Design review of the part built by this model. Coordinates are the model's own, in mm. Face numbers are marked on the shaded views. A direction names the side the tool comes from. Coordinates: 2 decimals unless noted, no trailing zeros. Loops run counter-clockwise (first coordinate to the right, second up) from the corner with the lowest first, then second, coordinate; pieces in that order, holes last. Notation, with made-up numbers: (84, 47) - (112, 47) arc R27 cw to (112, 64) - close; hole circle Ø2 at (37, 54). An arc over 180 degrees is marked (long way). Answer in a Markdown table with one row per item. Add a question column.
(1) The part is to be moulded in two halves that separate along X. For the marked faces 3, 4 and 5, say which applies: released by +X, released by -X, zero draft, split by the parting line, or undercut.
(2) We need section D-D, the plane x = 1. Write out the cut boundary in (y, z).
(3) We need section A-A, the plane x = 0. Write out the cut boundary in (y, z).
(4) For the marked faces 1 and 2, list the 3-axis set-ups (+Z, -Z, +X, -X, +Y, -Y) from which the entire face can be reached by the end or side of a thin tool; tool diameter is ignored.
(5) Clearance check with flat-ended pins moving along their axes: pin 1 (2.5 mm diameter, centred on x = 1, y = -0.5, fed in from -Z); pin 2 (2 mm diameter, centred on x = 3.5, z = 3, fed in from +Y); pin 3 (1 mm diameter, centred on x = 2.5, z = 1, fed in from +Y). State where each tip first meets the part, or that it passes through.
(6) We need section B-B, the plane y = 0. Write out the cut boundary in (x, z).
(7) To check wall thickness, follow L1, parallel to Y at x = 0, z = 2.2; L2, parallel to Y at x = 0, z = 3.85; L3, parallel to X at y = 0, z = 1.4. State the ranges of each line that lie inside material, in increasing order. Write a range as [from, to].
(8) We need section C-C, the plane z = 3.75. Write out the cut boundary in (x, y).
from build123d import *

# Parameters (mm, degrees)
F0_R     = 4.75
F1_DEPTH = 4
F2_R     = 2
F3_DEPTH = 4
F5_START = -0.75
F4_R     = 2.5
F5_DEPTH = 3.25
F6_W     = 3.7872615503
F6_H     = 0.8450912428
F7_DEPTH = 4


with BuildPart() as f1:
    # F0 (on Top) → F1 (new body)
    with BuildSketch(Plane.XY):
        Circle(F0_R)
    extrude(amount=F1_DEPTH)

    # F2 (on face) → F3 (cut)
    with BuildSketch(Plane.XY.offset(4)):
        Circle(F2_R)
    extrude(amount=-F3_DEPTH, mode=Mode.SUBTRACT)

    # F4 (on face) → F5 (cut)
    with BuildSketch(Plane.XY.offset(4).offset(F5_START)):
        Circle(F4_R)
    extrude(amount=-F5_DEPTH, mode=Mode.SUBTRACT)

    # F6 (on face) → F7 (cut)
    with BuildSketch(Plane.XY.offset(4)):
        with Locations((3.3074248931, -0.0251903548)):
            Rectangle(F6_W, F6_H)
    extrude(amount=-F7_DEPTH, mode=Mode.SUBTRACT)


solid = f1.part
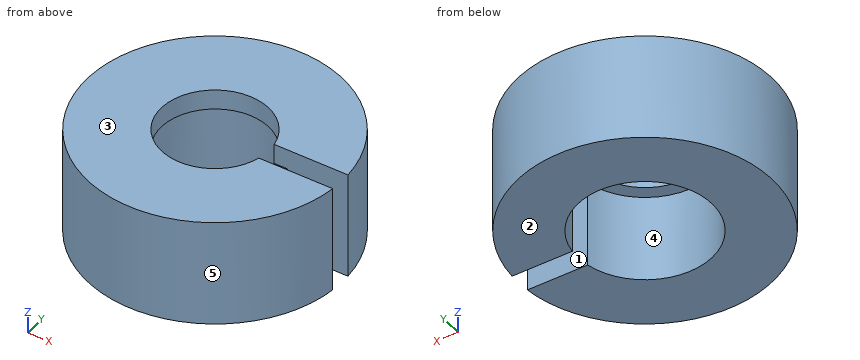
Responses:
| question | item | result |
|---|---|---|
| 1 | face 3 | zero draft |
| 1 | face 4 | undercut |
| 1 | face 5 | split by the parting line |
| 2 | outline | (-4.64, 0) - (-2.29, 0) - (-2.29, 3.25) - (-1.73, 3.25) - (-1.73, 4) - (-4.64, 4) - close; (1.73, 3.25) - (2.29, 3.25) - (2.29, 0) - (4.64, 0) - (4.64, 4) - (1.73, 4) - close |
| 3 | outline | (-4.75, 0) - (-2.5, 0) - (-2.5, 3.25) - (-2, 3.25) - (-2, 4) - (-4.75, 4) - close; (2, 3.25) - (2.5, 3.25) - (2.5, 0) - (4.75, 0) - (4.75, 4) - (2, 4) - close |
| 4 | face 1 | +Z, -Z, +X |
| 4 | face 2 | -Z, +X, -X, +Y, -Y |
| 5 | pin 1 | stops at z = 3.25 |
| 5 | pin 2 | stops at y = 4.04 |
| 5 | pin 3 | stops at y = 4.31 |
| 6 | outline | (-4.75, 0) - (-2.5, 0) - (-2.5, 3.25) - (-2, 3.25) - (-2, 4) - (-4.75, 4) - close |
| 7 | L1 | y = [-4.75, -2.5], [2.5, 4.75] |
| 7 | L2 | y = [-4.75, -2], [2, 4.75] |
| 7 | L3 | x = [-4.75, -2.5] |
| 8 | outline | (1.95, -0.45) arc R2 cw (long way) to (1.96, 0.4) - (4.73, 0.4) arc R4.75 ccw (long way) to (4.73, -0.45) - close |
